from build123d import *

# Parameters (mm, degrees)
F0_W     = 35
F0_H     = 8
F1_DEPTH = 2
F2_SIZE2 = 3.99999
F2_SIZE  = 1.99999
F3_W     = 4
F3_H     = 6.5
F4_DEPTH = 2
F5_W     = 10
F5_H     = 1.25
F6_DEPTH = 2


# Not quite as in the source:
# - a fillet or chamfer is up to 0.001 mm smaller than in the source, because OpenCascade refuses the exact size


with BuildPart() as f1:
    # F0 (on Front) → F1 (new body)
    with BuildSketch(Plane.XZ):
        with Locations((-17.5, 4)):
            Rectangle(F0_W, F0_H)
    extrude(amount=F1_DEPTH)

    # F2 (size 2 and 4 in the source; OpenCascade refuses exactly that, so slightly less here)
    f2_edges = [f1.edges().sort_by_distance(p)[0] for p in [
        (-35, -2, 4),
    ]]
    f2_side = f1.faces().sort_by_distance((-35, -1, 4))[0]
    chamfer(f2_edges, length=F2_SIZE, length2=F2_SIZE2, reference=f2_side)

    # F3 (on face) → F4 (cut)
    with BuildSketch(Plane.XZ.offset(2)):
        with Locations((-4, 4)):
            Rectangle(F3_W, F3_H)
    extrude(amount=-F4_DEPTH, mode=Mode.SUBTRACT)

    # F5 (on face) → F6 (cut)
    with BuildSketch(Plane.XZ.offset(2)):
        with Locations((-24, 4)):
            Rectangle(F5_W, F5_H)
    extrude(amount=-F6_DEPTH, mode=Mode.SUBTRACT)


solid = f1.part
The model under review builds one solid part; all positions refer to its coordinate system, in mm. A direction names the side the tool comes from. Round coordinates to 2 decimals unless told otherwise and drop trailing zeros. Loops run counter-clockwise (first coordinate to the right, second up) from the corner with the lowest first, then second, coordinate; pieces in that order, holes last. Notation, with made-up numbers: M 83.25,79 L 106.25,79 A30 cw 106.25,104 Z; hole C 12.5,-28 d4. An arc over 180 degrees is marked long. Answer as a JSON object with one key per item and string values.
Item 1: We need section C-C, the plane y = -1.6. State the section outline as (x, z) points (3 decimals).
Check sheet entries:
{"outline": "M -31.8,0 L 0,0 L 0,8 L -31.8,8 Z; hole M -29,3.375 L -19,3.375 L -19,4.625 L -29,4.625 Z; hole M -6,0.75 L -2,0.75 L -2,7.25 L -6,7.25 Z"}
Item 2: We need section D-D, the plane x = -5.5. State the section outline as (y, z) points.
Check sheet entries:
{"outline": "M -2,0 L 0,0 L 0,0.75 L -2,0.75 Z; M -2,7.25 L 0,7.25 L 0,8 L -2,8 Z"}
Item 3: Clearance check with flat-ended pins moving along their axes: P1, Ø0.6, axis at y = -1, z = 4.5, coming from the -X side; P2, Ø1, axis at x = -24, y = -0.5, coming from the -Z side. State where each tip first meets the part, or that it passes through.
Check sheet entries:
{"P1": "x = -33.6", "P2": "z = 0"}
Item 4: The part is to be moulded in two halves that separate along Z. For faces 1 (the face through (0, -1, 4)), 2 (the face through (-18, -1, 0)), 3 (the face through (-24, -1, 4.625)), 4 (the face through (-6, -1, 4)), say which applies: +Z half, -Z half, draft (parallel to the pull), parting line (faces both ways), or undercut.
Check sheet entries:
{"face 1": "draft", "face 2": "-Z half", "face 3": "undercut", "face 4": "undercut"}
Item 5: We need section A-A, the plane x = -22.5. State the section outline as (y, z) points (3 decimals), and give its area (3 significant figures).
Check sheet entries:
{"outline": "M -2,0 L 0,0 L 0,3.375 L -2,3.375 Z; M -2,4.625 L 0,4.625 L 0,8 L -2,8 Z", "area": "13.5 mm2"}
Item 6: For line 1 along Z through (x, y) = (-25, -0.7) (3 decimals); line 2 along X through (y, z) = (-1.15, 4); line 3 along X through (y, z) = (-0.25, 4.5), list the stretches that pass through material, from the lowest coordinate up.
Check sheet entries:
{"line 1": "0 to 3.375, 4.625 to 8", "line 2": "-32.7 to -29, -19 to -6, -2 to 0", "line 3": "-34.5 to -29, -19 to -6, -2 to 0"}
Item 7: Tool access review of faces 5 (the face through (-16, -2, 4)), 6 (the face through (-19, -1, 4)): name each direction out of +Z, -Z, +X, -X, +Y, -Y from which nothing blocks a thin tool from reaching the whole face with its end or side.
Check sheet entries:
{"face 5": "+Z, -Z, +X, -X, -Y", "face 6": "+Y, -Y"}
